Answer from the drawing. Dimensions are ordinates in mm from the lowest x, y and z of the part. A direction names the side the tool comes from. Coordinates: 2 decimals unless noted, no trailing zeros. Write each loop counter-clockwise with the first axis right and the second up, starting at its lowest first coordinate (ties: lowest second). Pieces come first, ordered by that corner, then holes. Notation, with made-up numbers: (6.25, 88.25) -> (37.25, 88.25) arc R28 cw to (37.25, 107.25) -> close; hole circle Ø9 at (22, 6.25). An arc over 180 degrees is marked (long way). Return JSON: item names as keys, results as strings.
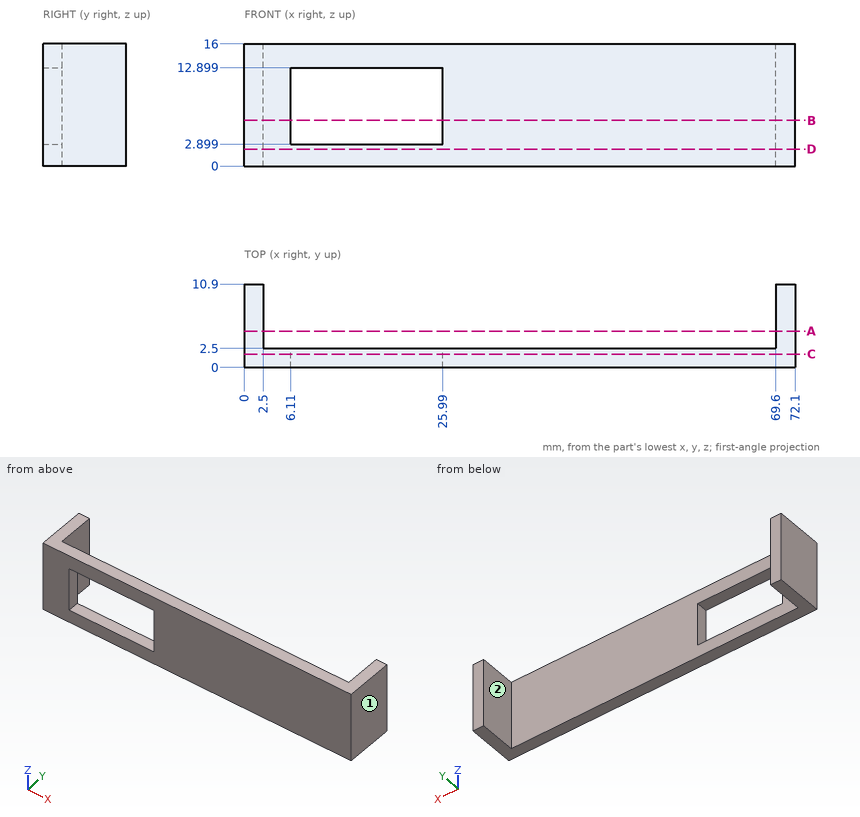
1. Flat-ended cylindrical pins translate along their axes: pin 1 Ø4 at (y, z) = (8, 10.5) entering from -X; pin 2 Ø5 at (x, z) = (28.5, 7) entering from +Y. Find the tip coordinate at first contact, or state that the pin passes through.
Taken from the geometry:
{"pin 1": "stops at x = 0", "pin 2": "stops at y = 2.5"}
2. The part is cut by section D-D (z = 2.25). Determine the outline of the cut face in (x, y).
Taken from the geometry:
{"outline": "(0, 0) -> (72.1, 0) -> (72.1, 10.9) -> (69.6, 10.9) -> (69.6, 2.5) -> (2.5, 2.5) -> (2.5, 10.9) -> (0, 10.9) -> close"}
3. Consider L1, parallel to Z at x = 13, y = 1.75; L2, parallel to X at y = 6.25, z = 2.75; L3, parallel to X at y = 2, z = 8. Determine where each line is inside the solid, lowest interval first.
Taken from the geometry:
{"L1": "z = 0 to 2.9, 12.9 to 16", "L2": "x = 0 to 2.5, 69.6 to 72.1", "L3": "x = 0 to 6.11, 25.99 to 72.1"}
4. A tool of negligible diameter and unlimited length cuts with its end or side. For the marked faces 1 and 2, from which of +Z, -Z, +X, -X, +Y, -Y can it reach the whole face along a straight path? Write none if from no direction.
Taken from the geometry:
{"face 1": "+Z, -Z, +X, +Y, -Y", "face 2": "+Z, -Z, +Y"}
5. The part is cut by section C-C (y = 1.75). Determine the outline of the cut face in (x, z).
Taken from the geometry:
{"outline": "(0, 0) -> (72.1, 0) -> (72.1, 16) -> (0, 16) -> close; hole (6.11, 2.9) -> (25.99, 2.9) -> (25.99, 12.9) -> (6.11, 12.9) -> close"}
6. The part is cut by section A-A (y = 4.75). Determine the outline of the cut face in (x, z).
Taken from the geometry:
{"outline": "(0, 0) -> (2.5, 0) -> (2.5, 16) -> (0, 16) -> close; (69.6, 0) -> (72.1, 0) -> (72.1, 16) -> (69.6, 16) -> close"}
7. The part is cut by section B-B (z = 6). Determine the outline of the cut face in (x, y).
Taken from the geometry:
{"outline": "(0, 0) -> (6.11, 0) -> (6.11, 2.5) -> (2.5, 2.5) -> (2.5, 10.9) -> (0, 10.9) -> close; (25.99, 0) -> (72.1, 0) -> (72.1, 10.9) -> (69.6, 10.9) -> (69.6, 2.5) -> (25.99, 2.5) -> close"}
